Build history of the part. All positions in model axes, mm. Face numbers are marked on the shaded views. Give positions to 0.01 mm unless a question says otherwise; leave off trailing zeros. Write each loop counter-clockwise with the first axis right and the second up, starting at its lowest first coordinate (ties: lowest second). Pieces come first, ordered by that corner, then holes. Notation, with made-up numbers: (-20.5, -9.5) -> (-15.5, -9.5) arc R24 ccw to (-15.5, 19.5) -> close; hole circle Ø7 at (-24.5, 71). An arc over 180 degrees is marked (long way). Put each result on its own line as item: value. Start each with the question number.
Item 1: Slice it at D-D, the plane y = 33. List the corners of the cut face in (x, z), plus the area to 3 significant figures.
Item 2: Flat gauge pins, fed straight in: pin 1 Ø11.5 at (x, y) = (0, 33) entering from +Z; pin 2 Ø3 at (x, z) = (-9.5, -13) entering from +Y. Where does each tip first touch, or does it go through?
Item 3: Slice it at A-A, the plane y = -22. List the corners of the cut face in (x, z) (3 decimals), plus the area to 3 significant figures.
Item 4: Drill centre lines: line 1 along Y through (x, z) = (0, 22.75); line 2 along Z through (x, y) = (-6, -17.5); line 3 along Y through (x, z) = (0, -20.5). Where is each one in solid material? Low to high.
Item 5: Slice it at B-B, the plane x = 0. Give the number of separate pieces and of enclosed holes in the cut face, plus the area to 3 significant figures.
Item 6: Slice it at C-C, the plane y = -10. List the corners of the cut face in (x, z), plus the area to 3 significant figures.
Item 7: Two-plate mould, pull along Z, no slides. Class the marked faces 1, 2, 3 and 4: pulls with the +Z half, pulls with the -Z half, needs draft (parallel to the pull), parting line crosses it, or undercut.
```python
from build123d import *

# Parameters (mm, degrees)
BOSS_EXTRUDE1_DEPTH         = 28
SKETCH2_W                   = 32
SKETCH2_H                   = 74
CUT_EXTRUDE1_DEPTH          = 28
CHAMFER1_SIZE               = 2
HOLE1_D                     = 10
HOLE1_DEPTH                 = 12
HOLE1_CBORE_D               = 12
HOLE1_CBORE_DEPTH           = 4
M6_TAPPED_HOLE1_D           = 5
M6_TAPPED_HOLE1_DEPTH       = 27
M6_TAPPED_HOLE1_CSINK_D     = 6.05
M6_TAPPED_HOLE1_CSINK_ANGLE = 90
M6_TAPPED_HOLE1_TIP         = 1.502151548


with BuildPart() as part:
    # Sketch1 → Boss-Extrude1 (new, symmetric)
    with BuildSketch(Plane.XY):
        Polygon((-7.5, 42), (7.5, 42), (12.5, 3), (12.5, -42), (-12.5, -42), (-12.5, 3), align=None)
    extrude(amount=BOSS_EXTRUDE1_DEPTH, both=True)

    # Sketch2 → Cut-Extrude1 (cut, symmetric)
    with BuildSketch(Plane(origin=(0, 0, 0), x_dir=(0, 0, -1), z_dir=(1, 0, 0))):
        with Locations((0, 5)):
            Rectangle(SKETCH2_W, SKETCH2_H)
    extrude(amount=CUT_EXTRUDE1_DEPTH, both=True, mode=Mode.SUBTRACT)

    # Chamfer1
    chamfer1_edges = [part.edges().sort_by_distance(p)[0] for p in [
        (-12.5, -32, 0),
        (12.5, -32, 0),
    ]]
    chamfer(chamfer1_edges, length=CHAMFER1_SIZE)

    # Hole1
    with Locations(Plane.XY.offset(28)):
        with Locations((0, 33)):
            hole1 = CounterBoreHole(HOLE1_D / 2, HOLE1_CBORE_D / 2, HOLE1_CBORE_DEPTH, depth=HOLE1_DEPTH)

    # Mirror1: Hole1 across plane
    add(hole1.mirror(Plane.XY), mode=Mode.SUBTRACT)

    # M6 Tapped Hole1
    with Locations(Plane.XY.offset(28)):
        with Locations((0, -22)):
            CounterSinkHole(M6_TAPPED_HOLE1_D / 2, M6_TAPPED_HOLE1_CSINK_D / 2, depth=M6_TAPPED_HOLE1_DEPTH, counter_sink_angle=M6_TAPPED_HOLE1_CSINK_ANGLE)
            with Locations((0, 0, -(M6_TAPPED_HOLE1_DEPTH + M6_TAPPED_HOLE1_TIP / 2))):  # 118° drill point
                Cone(0, M6_TAPPED_HOLE1_D / 2, M6_TAPPED_HOLE1_TIP, mode=Mode.SUBTRACT)


solid = part.part
```
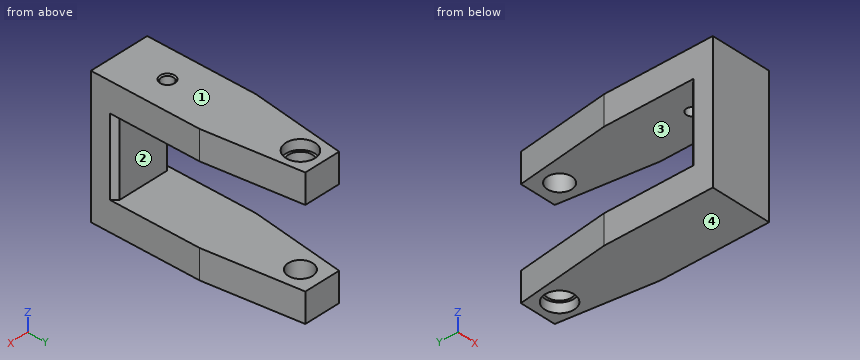
Values follow:
1. outline: (-8.65, -28) -> (-6, -28) -> (-6, -24) -> (-5, -24) -> (-5, -16) -> (-8.65, -16) -> close; (-8.65, 16) -> (-5, 16) -> (-5, 24) -> (-6, 24) -> (-6, 28) -> (-8.65, 28) -> close; (5, -24) -> (6, -24) -> (6, -28) -> (8.65, -28) -> (8.65, -16) -> (5, -16) -> close; (5, 16) -> (8.65, 16) -> (8.65, 28) -> (6, 28) -> (6, 24) -> (5, 24) -> close
1. area: 159 mm2
2. pin 1: z = 24
2. pin 2: y = -32
3. outline: (-12.5, -28) -> (12.5, -28) -> (12.5, -16) -> (-12.5, -16) -> close; (-12.5, 16) -> (-2.5, 16) -> (-2.5, 27.475) -> (-3.025, 28) -> (-12.5, 28) -> close; (2.5, 16) -> (12.5, 16) -> (12.5, 28) -> (3.025, 28) -> (2.5, 27.475) -> close
3. area: 540 mm2
4. line 1: -42 to -24.5, -19.5 to 28, 38 to 42
4. line 2: -28 to -16, 16 to 28
4. line 3: -42 to 28, 38 to 42
5. separate pieces: 4
5. enclosed holes: 0
5. area: 2,020 mm2
6. outline: (-12.5, -28) -> (12.5, -28) -> (12.5, -16) -> (-12.5, -16) -> close; (-12.5, 16) -> (12.5, 16) -> (12.5, 28) -> (-12.5, 28) -> close
6. area: 600 mm2
7. face 1: pulls with the +Z half
7. face 2: undercut
7. face 3: undercut
7. face 4: pulls with the -Z half
